```python
from build123d import *

# Parameters (mm, degrees)
F0_W      = 8
F0_H      = 18
F1_DEPTH  = 20
F2_R      = 1
F4_DEPTH  = 5
F6_DEPTH  = 2.5
F8_D      = 3.3
F8_DEPTH  = 10
F8_TIP    = 0.9914200214
F9_W      = 5.5
F9_H      = 2.5
F10_DEPTH = 7.35


with BuildPart() as f1:
    # F0 (on Front) → F1 (new body, symmetric)
    with BuildSketch(Plane.XZ):
        Polygon((-22.5, -2.5), (22.5, -2.5), (22.5, 2.5), (-14.5, 2.5), (-22.5, 2.5), align=None)
        with Locations((-18.5, 11.5)):
            Rectangle(F0_W, F0_H)
    extrude(amount=F1_DEPTH, both=True)

    # F2
    f2_edges = [f1.edges().sort_by_distance(p)[0] for p in [
        (-22.5, -20, 9),
        (-14.5, -20, 11.5),
        (22.5, -20, 0),
        (22.5, 20, 0),
        (-22.5, 20, 9),
        (-14.5, 20, 11.5),
    ]]
    fillet(f2_edges, radius=F2_R)

    # F3 (on face) → F4 (cut)
    with BuildSketch(Plane.XY.offset(2.5)):
        with BuildLine():
            ThreePointArc((-8.5, 11.65), (-10.15, 10), (-8.5, 8.35))
            Line((-8.5, 8.35), (16.5, 8.35))
            ThreePointArc((16.5, 8.35), (18.15, 10), (16.5, 11.65))
            Line((16.5, 11.65), (-8.5, 11.65))
        make_face()
        with BuildLine():
            ThreePointArc((-8.5, -8.35), (-10.15, -10), (-8.5, -11.65))
            Line((-8.5, -11.65), (16.5, -11.65))
            ThreePointArc((16.5, -11.65), (18.15, -10), (16.5, -8.35))
            Line((16.5, -8.35), (-8.5, -8.35))
        make_face()
    extrude(amount=-F4_DEPTH, mode=Mode.SUBTRACT)

    # F5 (on face) → F6 (cut)
    with BuildSketch(Plane.XY.offset(2.5)):
        with BuildLine():
            ThreePointArc((-8.5, 12.75), (-11.25, 10), (-8.5, 7.25))
            Line((-8.5, 7.25), (16.5, 7.25))
            ThreePointArc((16.5, 7.25), (19.25, 10), (16.5, 12.75))
            Line((16.5, 12.75), (-8.5, 12.75))
        make_face()
        with BuildLine():
            ThreePointArc((-8.5, -7.25), (-11.25, -10), (-8.5, -12.75))
            Line((-8.5, -12.75), (16.5, -12.75))
            ThreePointArc((16.5, -12.75), (19.25, -10), (16.5, -7.25))
            Line((16.5, -7.25), (-8.5, -7.25))
        make_face()
    extrude(amount=-F6_DEPTH, mode=Mode.SUBTRACT)

    # F8
    with Locations(Plane.XY.offset(20.5)):
        with Locations((-18.5, 10), (-18.5, -10)):
            Hole(F8_D / 2, depth=F8_DEPTH)
            with Locations((0, 0, -(F8_DEPTH + F8_TIP / 2))):  # 118° drill point
                Cone(0, F8_D / 2, F8_TIP, mode=Mode.SUBTRACT)

    # F9 (on face) → F10 (cut)
    with BuildSketch(Plane(origin=(-22.5, 0, 0), x_dir=(0, -1, 0), z_dir=(-1, 0, 0))):
        with Locations((-10, 15.5)):
            Rectangle(F9_W, F9_H)
        with Locations((10, 15.5)):
            Rectangle(F9_W, F9_H)
    extrude(amount=-F10_DEPTH, mode=Mode.SUBTRACT)


solid = f1.part
```
Can you work these out from the model? Positions are in its coordinate system, mm. A direction names the side the tool comes from. Round coordinates to 2 decimals unless told otherwise and drop trailing zeros. Loops run counter-clockwise (first coordinate to the right, second up) from the corner with the lowest first, then second, coordinate; pieces in that order, holes last.
Item 1: Suppose I cut it at D-D, the plane y = 9. State how many separate pieces and enclosed holes the cut face has, then the cut area to 3 significant figures.
Item 2: Suppose I cut it at C-C, the plane z = 7. Write out the boundary of the cut face in (x, y).
Item 3: Which directions (+Z, -Z, +X, -X, +Y, -Y) give clear straight access to the entire face, cutting with the end or side of a thin tool? Please do faces 1 (the flat face through (4, 8, 0)), 2 (the cylindrical face through (-10.15, -9.96, -1.23)), 3 (the flat face through (-15.15, -10, 16)), 4 (the cylindrical face through (-14.785, 19.699, 11.626)).
Item 4: Will these pins go through, and if not, where does the flat tip stop? pin 1 Ø5.5 at (y, z) = (-8, 10.5) entering from +X; pin 2 Ø3 at (x, y) = (8, -9.5) entering from +Z; pin 3 Ø2 at (x, y) = (-13, -13.5) entering from +Z.
Item 5: Suppose I cut it at A-A, the plane z = 1.5. Write out the boundary of the cut face in (x, y).
Item 6: If we mould it in two halves opening along X, with no side actions, what happens to faces 5 (the cylindrical face through (-22.215, -19.699, 8.839)), 6 (the flat face through (4, 12.75, 1)), 7 (the flat face through (-6, -20, 2))? For each: +X half, -X half, draft (parallel to the pull), parting line (faces both ways), or undercut.
Item 7: Suppose I cut it at B-B, the plane y = 2. Write out the boundary of the cut face in (x, z).
Item 8: Please list where these lines run through material, in increasing order: L1, parallel to Y at x = -7, z = -1; L2, parallel to X at y = -10, z = 1.25; L3, parallel to X at y = -10, z = 12.75.
Reported:
1. separate pieces: 3
1. enclosed holes: 0
1. area: 186 mm2
2. outline: (-22.5, -19) arc R1 ccw to (-21.5, -20) - (-15.5, -20) arc R1 ccw to (-14.5, -19) - (-14.5, 19) arc R1 ccw to (-15.5, 20) - (-21.5, 20) arc R1 ccw to (-22.5, 19) - close
3. face 1: +Z
3. face 2: +Z, -Z
3. face 3: -X
3. face 4: +Z, +X, +Y
4. pin 1: stops at x = -14.5
4. pin 2: stops at z = 0
4. pin 3: stops at z = 2.5
5. outline: (-22.5, -19) arc R1 ccw to (-21.5, -20) - (21.5, -20) arc R1 ccw to (22.5, -19) - (22.5, 19) arc R1 ccw to (21.5, 20) - (-21.5, 20) arc R1 ccw to (-22.5, 19) - close; hole (-8.5, -12.75) - (16.5, -12.75) arc R2.75 ccw to (16.5, -7.25) - (-8.5, -7.25) arc R2.75 ccw to start; hole (-8.5, 7.25) - (16.5, 7.25) arc R2.75 ccw to (16.5, 12.75) - (-8.5, 12.75) arc R2.75 ccw to start
6. face 5: -X half
6. face 6: undercut
6. face 7: draft
7. outline: (-22.5, -2.5) - (22.5, -2.5) - (22.5, 2.5) - (-14.5, 2.5) - (-14.5, 20.5) - (-22.5, 20.5) - close
8. L1: y = -20 to -11.65, -8.35 to 8.35, 11.65 to 20
8. L2: x = -22.5 to -11.25, 19.25 to 22.5
8. L3: x = -22.5 to -20.15, -16.85 to -14.5
